Job drawing, mm, ordinate dimensions from the low corner. One solid piece. A direction names the side the tool comes from. Give positions to 0.01 mm unless a question says otherwise; leave off trailing zeros. Loops run counter-clockwise (first coordinate to the right, second up) from the corner with the lowest first, then second, coordinate; pieces in that order, holes last. Notation, with made-up numbers: M 77,36.25 L 128,36.25 A23 ccw 128,66.25 Z; hole C 40,-17 d3. An arc over 180 degrees is marked long. Put each result on its own line as item: value.
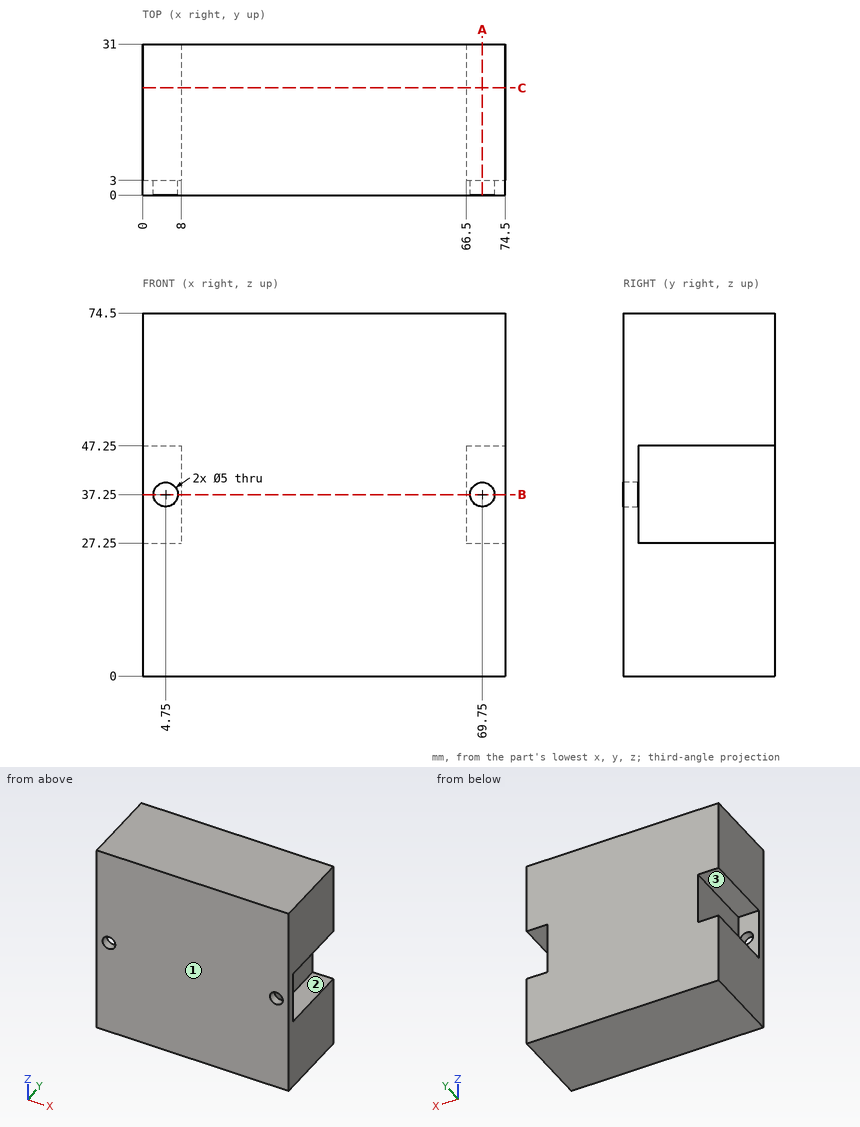
Q1. Probe line 1 (X direction, y = 1, z = 37); line 2 (Z direction, x = 4.75, y = 1.15); line 3 (X direction, y = 26, z = 35). List the from-to ranges inside material, lowest first. Write a range as from..to.
Here are the results:
line 1: 0..2.26, 7.24..67.26, 72.24..74.5
line 2: 0..34.75, 39.75..74.5
line 3: 8..66.5
Q2. Slice it at A-A (x = 69.75). List the corners of the cut face in (y, z).
Here are the results:
outline: M 0,0 L 31,0 L 31,27.25 L 3,27.25 L 3,34.75 L 0,34.75 Z; M 0,39.75 L 3,39.75 L 3,47.25 L 31,47.25 L 31,74.5 L 0,74.5 Z
Q3. Drop flat-ended pins along their axis: pin 1 Ø6 at (y, z) = (23.5, 36.5) entering from -X; pin 2 Ø2.5 at (x, z) = (2.5, 39.5) entering from +Y. Give the stop position or say it passes through.
Here are the results:
pin 1: x = 8
pin 2: y = 3
Q4. Slice it at C-C (y = 22). List the corners of the cut face in (x, z).
Here are the results:
outline: M 0,0 L 74.5,0 L 74.5,27.25 L 66.5,27.25 L 66.5,47.25 L 74.5,47.25 L 74.5,74.5 L 0,74.5 L 0,47.25 L 8,47.25 L 8,27.25 L 0,27.25 Z
Q5. Tool access for the marked faces 1, 2 and 3: list every direction of +Z, -Z, +X, -X, +Y, -Y with a clear straight run to the whole face (end or side of a thin tool).
Here are the results:
face 1: +Z, -Z, +X, -X, -Y
face 2: +X, +Y
face 3: -X, +Y
Q6. Slice it at B-B (z = 37.25). List the corners of the cut face in (x, y), and give its area (3 significant figures).
Here are the results:
outline: M 0,0 L 2.25,0 L 2.25,3 L 0,3 Z; M 7.25,0 L 67.25,0 L 67.25,3 L 66.5,3 L 66.5,31 L 8,31 L 8,3 L 7.25,3 Z; M 72.25,0 L 74.5,0 L 74.5,3 L 72.25,3 Z
area: 1,830 mm²
